Read the model definition and answer for the solid it produces. Units are mm, in the model's axes. Face numbers are marked on the shaded views. A direction names the side the tool comes from. Coordinates: 2 decimals unless noted, no trailing zeros. Order: outer loops, then holes, each group sorted by start corner. A loop starts at its lowest first (then second) coordinate and runs counter-clockwise, first axis right, second up. Notation, with made-up numbers: (60.25, 58) -> (90.25, 58) arc R20 cw to (90.25, 89) -> close; hole circle Ø5 at (-17.5, 14.25). An arc over 180 degrees is marked (long way). Answer in a Markdown table with one row per item.
from build123d import *

# Parameters (mm, degrees)
F2_SIZE = 1
F3_SIZE = 2
F4_R    = 2.2
F6_D    = 3.3


with BuildPart() as f1:
    # F0 (on Top) → F1 (revolve)
    with BuildSketch(Plane.XY):
        Polygon((-20.039994, 3), (-20.039994, 0), (-1.039994, 0), (-1.039994, 3), (-4.039994, 3), (-4.039994, 8), (-1.039994, 8), (-1.039994, 13), (-8.039994, 13), (-8.039994, 8), (-13.039994, 8), (-13.039994, 13), (-20.039994, 13), (-20.039994, 8), (-17.039994, 8), (-17.039994, 3), align=None)
    revolve(axis=Axis((-10.68385, 0, 0), (1, 0, 0)))

    # F2
    f2_edges = [f1.edges().sort_by_distance(p)[0] for p in [
        (-1.039994, -8, 0),
        (-20.039994, -8, 0),
    ]]
    chamfer(f2_edges, length=F2_SIZE)

    # F3
    f3_edges = [f1.edges().sort_by_distance(p)[0] for p in [
        (-20.039994, -13, 0),
        (-1.039994, -13, 0),
    ]]
    chamfer(f3_edges, length=F3_SIZE)

    # F4
    f4_edges = [f1.edges().sort_by_distance(p)[0] for p in [
        (-13.039994, -8, 0),
        (-8.039994, -8, 0),
    ]]
    fillet(f4_edges, radius=F4_R)

    # F6 (through all)
    with Locations(Plane(origin=(-20.039994, 0, 0), x_dir=(0, -1, 0), z_dir=(-1, 0, 0))):
        with Locations((0, 0)):
            Hole(F6_D / 2)


solid = f1.part
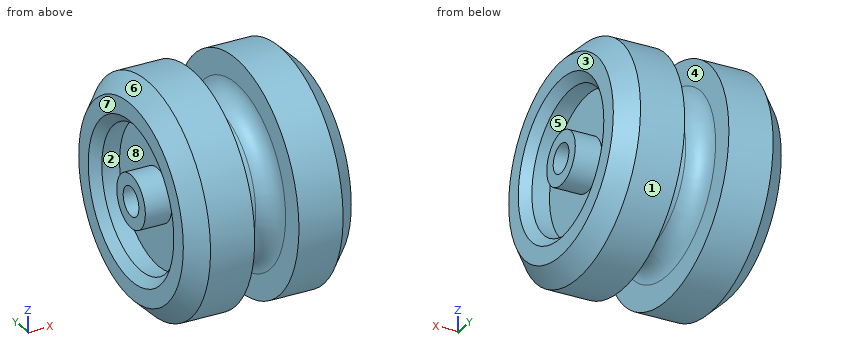
Q1. The part is cut by section A-A (x = -6.5). Write down the section's boundary in (y, z), then the cut area to 3 significant figures.
Outcome:
| item | result |
|---|---|
| outline | circle Ø26 at (0, 0); hole circle Ø3.3 at (0, 0) |
| area | 522 mm² |
Q2. Consider line 1 (Z direction, x = -17.5, y = 0); line 2 (X direction, y = 7.75, z = 1.5); line 3 (X direction, y = -10.75, z = -1.75). Determine where each line is inside the solid, lowest interval first.
Outcome:
| item | result |
|---|---|
| line 1 | -13 to -8, -3 to -1.65, 1.65 to 3, 8 to 13 |
| line 2 | -17.04 to -4.04 |
| line 3 | -20.04 to -13.04, -8.04 to -1.04 |
Q3. Given pin 1 (8 mm diameter, centred on x = -7.5, y = 8.5, fed in from +Z); pin 2 (2 mm diameter, centred on x = -6.5, z = 10, fed in from -Y); pin 3 (5 mm diameter, centred on x = -12.5, y = -4, fed in from +Z); pin 4 (2.5 mm diameter, centred on y = 0, z = 0, fed in from +X), each flat-ended and moving along its own axis, determine where each tip first touches the part or whether it passes through.
Outcome:
| item | result |
|---|---|
| pin 1 | z = 12.2 |
| pin 2 | y = -9.38 |
| pin 3 | z = 12.91 |
| pin 4 | through |
Q4. For a pull along Y with two mould halves and no side action, classify the marked faces 6, 7 and 8 as pulls with the +Y half, pulls with the -Y half, needs draft (parallel to the pull), parting line crosses it, or undercut.
Outcome:
| item | result |
|---|---|
| face 6 | parting line crosses it |
| face 7 | needs draft |
| face 8 | undercut |
Q5. For the marked faces 1, 2, 3, 4 and 5, determine the directions among +Z, -Z, +X, -X, +Y, -Y from which every point of the face is accessible in a straight line to the end or side of a thin tool.
Outcome:
| item | result |
|---|---|
| face 1 | +X, -X |
| face 2 | -X |
| face 3 | +Z, -Z, +X, +Y, -Y |
| face 4 | none |
| face 5 | +X |
